from build123d import *

# Parameters (mm, degrees)
SKETCH1_W          = 20.701
SKETCH1_H          = 6.223
EXTRUDE1_DEPTH     = 8.636
CUT_EXTRUDE1_DEPTH = 25.4
CUT_EXTRUDE2_DEPTH = 25.4
SKETCH4_R          = 1.016
CUT_EXTRUDE3_DEPTH = 0.508
CUT_EXTRUDE4_DEPTH = 0.508
SKETCH6_W          = 1.82195604
SKETCH6_H          = 3.576432228
CUT_EXTRUDE5_DEPTH = 1.27
CHAMFER1_SIZE      = 0.508
SKETCH7_W          = 0.80595604
SKETCH7_H          = 0.757943843
CUT_EXTRUDE6_DEPTH = 1.27
SKETCH8_W          = 0.433382436
SKETCH8_H          = 0.491166761
EXTRUDE2_DEPTH     = 1.905
SKETCH9_W          = 13.835725518
SKETCH9_H          = 11.068580414
CUT_EXTRUDE7_DEPTH = 25.4
SKETCH10_W         = 3.388588983
SKETCH10_H         = 10.514703946
CUT_EXTRUDE8_DEPTH = 25.4


with BuildPart() as part:
    # Sketch1 → Extrude1 (new body)
    with BuildSketch(Plane(origin=(0, 0, 0), x_dir=(1, 0, 0), z_dir=(0, 1, 0))):
        with Locations((10.3505, 3.1115)):
            Rectangle(SKETCH1_W, SKETCH1_H)
    extrude(amount=EXTRUDE1_DEPTH)

    # Sketch2 → Cut-Extrude1 (cut)
    with BuildSketch(Plane(origin=(20.701, 0, 0), x_dir=(0, 0, -1), z_dir=(1, 0, 0))):
        Polygon((-2.869110069, 4.645946632), (0.62179162, 4.645946632), (2.217632392, 11.827230107), (-2.869110069, 11.827230107), align=None)
    extrude(amount=-CUT_EXTRUDE1_DEPTH, mode=Mode.SUBTRACT)

    # Sketch3 → Cut-Extrude2 (cut)
    with BuildSketch(Plane(origin=(20.701, 0, 0), x_dir=(0, 0, -1), z_dir=(1, 0, 0))):
        Polygon((4.012953261, 10.231389335), (6.905414661, 0.855824797), (9.199435771, 0.855824797), (9.199435771, 10.231389335), align=None)
    extrude(amount=-CUT_EXTRUDE2_DEPTH, mode=Mode.SUBTRACT)

    # Sketch4 → Cut-Extrude3 (cut)
    with BuildSketch(Plane(origin=(0, 8.636, 0), x_dir=(1, 0, 0), z_dir=(0, 1, 0))):
        with Locations((1.27, 2.949100672)):
            Circle(SKETCH4_R)
        with Locations((3.81, 2.949100672)):
            Circle(SKETCH4_R)
        with Locations((6.35, 2.949100672)):
            Circle(SKETCH4_R)
        with Locations((8.89, 2.949100672)):
            Circle(SKETCH4_R)
        with Locations((11.43, 2.949100672)):
            Circle(SKETCH4_R)
        with Locations((13.97, 2.949100672)):
            Circle(SKETCH4_R)
        with Locations((16.51, 2.949100672)):
            Circle(SKETCH4_R)
        with Locations((19.05, 2.949100672)):
            Circle(SKETCH4_R)
    extrude(amount=-CUT_EXTRUDE3_DEPTH, mode=Mode.SUBTRACT)

    # Sketch5 → Cut-Extrude4 (cut)
    with BuildSketch(Plane(origin=(0, 8.128, 0), x_dir=(1, 0, 0), z_dir=(0, 1, 0))):
        with BuildLine():
            ThreePointArc((0.55685802, 3.67276117), (0.471993814, 3.577942566), (0.399647546, 3.473259623))
            Line((0.399647546, 3.473259623), (1.98314198, 2.225440174))
            ThreePointArc((1.98314198, 2.225440174), (2.068006186, 2.320258778), (2.140352454, 2.42494172))
            Line((2.140352454, 2.42494172), (0.55685802, 3.67276117))
        make_face()
        with BuildLine():
            ThreePointArc((2.939647546, 2.42494172), (3.011993814, 2.320258778), (3.09685802, 2.225440174))
            Line((3.09685802, 2.225440174), (4.680352454, 3.473259623))
            ThreePointArc((4.680352454, 3.473259623), (4.608006186, 3.577942566), (4.52314198, 3.67276117))
            Line((4.52314198, 3.67276117), (2.939647546, 2.42494172))
        make_face()
        with BuildLine():
            ThreePointArc((5.34196875, 3.076100672), (5.334, 2.949100672), (5.34196875, 2.822100672))
            Line((5.34196875, 2.822100672), (7.35803125, 2.822100672))
            ThreePointArc((7.35803125, 2.822100672), (7.364005855, 2.885475793), (7.366, 2.949100672))
            ThreePointArc((7.366, 2.949100672), (7.364005855, 3.012725551), (7.35803125, 3.076100672))
            Line((7.35803125, 3.076100672), (5.34196875, 3.076100672))
        make_face()
        with BuildLine():
            ThreePointArc((8.458529789, 2.041483422), (8.576688012, 1.994233554), (8.699870069, 1.9622946))
            Line((8.699870069, 1.9622946), (9.321470211, 3.856717921))
            ThreePointArc((9.321470211, 3.856717921), (9.203311988, 3.90396779), (9.080129931, 3.935906744))
            Line((9.080129931, 3.935906744), (8.458529789, 2.041483422))
        make_face()
        with BuildLine():
            ThreePointArc((11.557, 3.957131921), (11.43, 3.965100672), (11.303, 3.957131921))
            Line((11.303, 3.957131921), (11.303, 1.941069422))
            ThreePointArc((11.303, 1.941069422), (11.43, 1.933100672), (11.557, 1.941069422))
            Line((11.557, 1.941069422), (11.557, 3.957131921))
        make_face()
        with BuildLine():
            ThreePointArc((13.060727808, 3.402399778), (13.011197076, 3.285185412), (12.976706622, 3.162699047))
            Line((12.976706622, 3.162699047), (14.879272192, 2.495801565))
            ThreePointArc((14.879272192, 2.495801565), (14.928802924, 2.613015931), (14.963293378, 2.735502296))
            Line((14.963293378, 2.735502296), (13.060727808, 3.402399778))
        make_face()
        with BuildLine():
            ThreePointArc((16.944941036, 3.867295801), (16.826755289, 3.914461789), (16.703600756, 3.946484624))
            Line((16.703600756, 3.946484624), (16.075058964, 2.030905542))
            ThreePointArc((16.075058964, 2.030905542), (16.193244711, 1.983739555), (16.316399244, 1.95171672))
            Line((16.316399244, 1.95171672), (16.944941036, 3.867295801))
        make_face()
        with BuildLine():
            ThreePointArc((18.349819557, 3.662547267), (18.264852019, 3.567810091), (18.192609083, 3.463045721))
            Line((18.192609083, 3.463045721), (19.750180443, 2.235654077))
            ThreePointArc((19.750180443, 2.235654077), (19.835147981, 2.330391253), (19.907390917, 2.435155623))
            Line((19.907390917, 2.435155623), (18.349819557, 3.662547267))
        make_face()
    extrude(amount=-CUT_EXTRUDE4_DEPTH, mode=Mode.SUBTRACT)

    # Sketch6 → Cut-Extrude5 (cut)
    with BuildSketch(Plane.XY):
        with Locations((3.861070401, 2.24061075)):
            Rectangle(SKETCH6_W, SKETCH6_H)
        with Locations((1.321070401, 2.24061075)):
            Rectangle(SKETCH6_W, SKETCH6_H)
        with Locations((6.401070401, 2.24061075)):
            Rectangle(SKETCH6_W, SKETCH6_H)
        with Locations((8.941070401, 2.24061075)):
            Rectangle(SKETCH6_W, SKETCH6_H)
        with Locations((11.481070401, 2.24061075)):
            Rectangle(SKETCH6_W, SKETCH6_H)
        with Locations((14.021070401, 2.24061075)):
            Rectangle(SKETCH6_W, SKETCH6_H)
        with Locations((16.561070401, 2.24061075)):
            Rectangle(SKETCH6_W, SKETCH6_H)
        with Locations((19.101070401, 2.24061075)):
            Rectangle(SKETCH6_W, SKETCH6_H)
    extrude(amount=-CUT_EXTRUDE5_DEPTH, mode=Mode.SUBTRACT)

    # Chamfer1
    chamfer1_edges = [part.edges().sort_by_distance(p)[0] for p in [
        (0.410092381, 2.24061075, -1.27),
        (1.321070401, 4.028826864, -1.27),
        (2.232048421, 2.24061075, -1.27),
        (1.321070401, 0.452394636, -1.27),
        (3.861070401, 4.028826864, -1.27),
        (4.772048421, 2.24061075, -1.27),
        (3.861070401, 0.452394636, -1.27),
        (2.950092381, 2.24061075, -1.27),
        (6.401070401, 4.028826864, -1.27),
        (7.312048421, 2.24061075, -1.27),
        (6.401070401, 0.452394636, -1.27),
        (5.490092381, 2.24061075, -1.27),
        (8.941070401, 4.028826864, -1.27),
        (9.852048421, 2.24061075, -1.27),
        (8.941070401, 0.452394636, -1.27),
        (8.030092381, 2.24061075, -1.27),
        (11.481070401, 4.028826864, -1.27),
        (12.392048421, 2.24061075, -1.27),
        (11.481070401, 0.452394636, -1.27),
        (10.570092381, 2.24061075, -1.27),
        (14.021070401, 4.028826864, -1.27),
        (14.932048421, 2.24061075, -1.27),
        (14.021070401, 0.452394636, -1.27),
        (13.110092381, 2.24061075, -1.27),
        (16.561070401, 4.028826864, -1.27),
        (17.472048421, 2.24061075, -1.27),
        (16.561070401, 0.452394636, -1.27),
        (15.650092381, 2.24061075, -1.27),
        (19.101070401, 4.028826864, -1.27),
        (20.012048421, 2.24061075, -1.27),
        (19.101070401, 0.452394636, -1.27),
        (18.190092381, 2.24061075, -1.27),
    ]]
    chamfer(chamfer1_edges, length=CHAMFER1_SIZE)

    # Sketch7 → Cut-Extrude6 (cut)
    with BuildSketch(Plane.XY.offset(-1.27)):
        with Locations((1.321070401, 2.17271271)):
            Rectangle(SKETCH7_W, SKETCH7_H)
        with Locations((3.861070401, 2.17271271)):
            Rectangle(SKETCH7_W, SKETCH7_H)
        with Locations((6.401070401, 2.17271271)):
            Rectangle(SKETCH7_W, SKETCH7_H)
        with Locations((8.941070401, 2.17271271)):
            Rectangle(SKETCH7_W, SKETCH7_H)
        with Locations((11.481070401, 2.17271271)):
            Rectangle(SKETCH7_W, SKETCH7_H)
        with Locations((14.021070401, 2.17271271)):
            Rectangle(SKETCH7_W, SKETCH7_H)
        with Locations((16.561070401, 2.17271271)):
            Rectangle(SKETCH7_W, SKETCH7_H)
        with Locations((19.101070401, 2.17271271)):
            Rectangle(SKETCH7_W, SKETCH7_H)
    extrude(amount=-CUT_EXTRUDE6_DEPTH, mode=Mode.SUBTRACT)

    # Sketch8 → Extrude2 (add)
    with BuildSketch(Plane.XZ):
        with Locations((3.829530977, -2.990246105)):
            Rectangle(SKETCH8_W, SKETCH8_H)
        with Locations((1.289530977, -2.990246105)):
            Rectangle(SKETCH8_W, SKETCH8_H)
        with Locations((6.369530977, -2.990246105)):
            Rectangle(SKETCH8_W, SKETCH8_H)
        with Locations((8.909530977, -2.990246105)):
            Rectangle(SKETCH8_W, SKETCH8_H)
        with Locations((11.449530977, -2.990246105)):
            Rectangle(SKETCH8_W, SKETCH8_H)
        with Locations((13.989530977, -2.990246105)):
            Rectangle(SKETCH8_W, SKETCH8_H)
        with Locations((16.529530977, -2.990246105)):
            Rectangle(SKETCH8_W, SKETCH8_H)
        with Locations((19.069530977, -2.990246105)):
            Rectangle(SKETCH8_W, SKETCH8_H)
    extrude(amount=EXTRUDE2_DEPTH)

    # Sketch9 → Cut-Extrude7 (cut)
    with BuildSketch(Plane(origin=(0, 8.636, 0), x_dir=(1, 0, 0), z_dir=(0, 1, 0))):
        with Locations((14.474610491, 2.472928053)):
            Rectangle(SKETCH9_W, SKETCH9_H)
    extrude(amount=-CUT_EXTRUDE7_DEPTH, mode=Mode.SUBTRACT)

    # Sketch10 → Cut-Extrude8 (cut)
    with BuildSketch(Plane(origin=(0, 8.636, 0), x_dir=(1, 0, 0), z_dir=(0, 1, 0))):
        with Locations((6.914242224, 3.1115)):
            Rectangle(SKETCH10_W, SKETCH10_H)
    extrude(amount=-CUT_EXTRUDE8_DEPTH, mode=Mode.SUBTRACT)


solid = part.part
Verification items for the finished model (mm, model axes). A direction names the side the tool comes from. Round coordinates to 2 decimals unless told otherwise and drop trailing zeros. Loops run counter-clockwise (first coordinate to the right, second up) from the corner with the lowest first, then second, coordinate; pieces in that order, holes last. Notation, with made-up numbers: M 17.25,-17.5 L 47.25,-17.5 A30 ccw 47.25,18.5 Z; hole C 3.5,6.25 d5. An arc over 180 degrees is marked long. Write each question's results on one line, items separated by ' | '.
1) Section check A-A on y = -0.75. Record the boundary of the cut face in (x, z), then the cut area to 3 significant figures.
Checks:
outline: M 1.07,-3.24 L 1.51,-3.24 L 1.51,-2.74 L 1.07,-2.74 Z; M 3.61,-3.24 L 4.05,-3.24 L 4.05,-2.74 L 3.61,-2.74 Z | area: 0.426 mm2
2) Section check B-B on y = 0.75. Record the boundary of the cut face in (x, z).
Checks:
outline: M 0,-6.22 L 5.22,-6.22 L 5.22,0 L 4.77,0 L 4.77,-0.76 L 4.47,-1.06 L 3.25,-1.06 L 2.95,-0.76 L 2.95,0 L 2.23,0 L 2.23,-0.76 L 1.93,-1.06 L 0.71,-1.06 L 0.41,-0.76 L 0.41,0 L 0,0 Z
3) Mould release check, pull along X, two halves, no side actions. Record for faces 1 (the flat face through (5.22, 4, -3)), 2 (the flat face through (4, 3, -1.27)), 3 (the flat face through (3, 2, -6.223)): released by +X, released by -X, zero draft, split by the parting line, or undercut.
Checks:
face 1: released by +X | face 2: undercut | face 3: zero draft
4) Section check D-D on y = 7.5. Record the boundary of the cut face in (x, z), then the cut area to 3 significant figures.
Checks:
outline: M 0,-4.86 L 5.22,-4.86 L 5.22,-1.26 L 0,-1.26 Z | area: 18.8 mm2
5) Gauge pin test, flat ends, axial feed: P1, Ø2, axis at x = 4, y = -0.5, coming from the +Z side; P2, Ø0.5, axis at y = -1.5, z = -3, coming from the +X side; P3, Ø0.5, axis at y = -1, z = -3, coming from the -X side; P4, Ø0.6, axis at x = 1, z = -0.5, coming from the -Y side. Record the tip position at first contact, or that the pin passes through.
Checks:
P1: stops at z = 0 | P2: stops at x = 4.05 | P3: stops at x = 1.07 | P4: stops at y = 0
6) Access from +Z, -Z, +X, -X, +Y, -Y to the whole of each face (thin tool, end or side, straight path). Record for faces 4 (the flat face through (4.1, 8.128, -2.5)), 5 (the flat face through (2.6, 8.636, -3)), 6 (the flat face through (4, 2.552, -2)).
Checks:
face 4: +Y | face 5: +Z, -Z, +X, -X, +Y | face 6: +Z
7) Scan lines: L1, parallel to Y at x = 4, z = -2.5; L2, parallel to Y at x = 2.45, z = -0.25; L3, parallel to Z at x = 3.81, y = 8.55. Record each from-to range of solid material in increasing order. Write a range as from..to.
Checks:
L1: y = 0..1.79, 2.55..8.13 | L2: y = 0..4.65 | L3: z = -4.53..-3.97, -1.93..-1.49
